```python
from build123d import *

# Parameters (mm, degrees)
CROQUIS1_R                        = 5.05
SALIENTE_EXTRUIR1_DEPTH           = 220
CORTAR_EXTRUIR1_REACH             = 7.05
CROQUIS2_R                        = 1.5
CORTAR_EXTRUIR1_DIRECTION_2_REACH = 7.05


with BuildPart() as part:
    # Croquis1 → Saliente-Extruir1 (new body)
    with BuildSketch(Plane(origin=(0, 0, 0), x_dir=(0, 0, -1), z_dir=(1, 0, 0))):
        Circle(CROQUIS1_R)
    extrude(amount=SALIENTE_EXTRUIR1_DEPTH)

    # Croquis2 → Cortar-Extruir1 (cut, up to next)
    with BuildSketch(Plane.XY, mode=Mode.PRIVATE) as cortar_extruir1_sk1:
        with Locations((3, 0)):
            Circle(CROQUIS2_R)
    cortar_extruir1_tool1 = extrude(cortar_extruir1_sk1.sketch, amount=-CORTAR_EXTRUIR1_REACH, mode=Mode.PRIVATE) & part.part
    add(cortar_extruir1_tool1.solids().sort_by_distance((3, 0, 0))[0], mode=Mode.SUBTRACT)
    # Croquis2 → Cortar-Extruir1 (cut, up to next)
    with BuildSketch(Plane.XY, mode=Mode.PRIVATE) as cortar_extruir1_sk2:
        with Locations((217, 0)):
            Circle(CROQUIS2_R)
    cortar_extruir1_tool2 = extrude(cortar_extruir1_sk2.sketch, amount=-CORTAR_EXTRUIR1_REACH, mode=Mode.PRIVATE) & part.part
    add(cortar_extruir1_tool2.solids().sort_by_distance((217, 0, 0))[0], mode=Mode.SUBTRACT)

    # Croquis2 → Cortar-Extruir1 direction 2 (cut, up to next)
    with BuildSketch(Plane.XY, mode=Mode.PRIVATE) as cortar_extruir1_direction_2_sk1:
        with Locations((3, 0)):
            Circle(CROQUIS2_R)
    cortar_extruir1_direction_2_tool1 = extrude(cortar_extruir1_direction_2_sk1.sketch, amount=CORTAR_EXTRUIR1_DIRECTION_2_REACH, mode=Mode.PRIVATE) & part.part
    add(cortar_extruir1_direction_2_tool1.solids().sort_by_distance((3, 0, 0))[0], mode=Mode.SUBTRACT)
    # Croquis2 → Cortar-Extruir1 direction 2 (cut, up to next)
    with BuildSketch(Plane.XY, mode=Mode.PRIVATE) as cortar_extruir1_direction_2_sk2:
        with Locations((217, 0)):
            Circle(CROQUIS2_R)
    cortar_extruir1_direction_2_tool2 = extrude(cortar_extruir1_direction_2_sk2.sketch, amount=CORTAR_EXTRUIR1_DIRECTION_2_REACH, mode=Mode.PRIVATE) & part.part
    add(cortar_extruir1_direction_2_tool2.solids().sort_by_distance((217, 0, 0))[0], mode=Mode.SUBTRACT)


solid = part.part
```
Geometry check sheet. Reference: the model listing, model coordinates, mm. Give positions to 0.01 mm unless a question says otherwise; leave off trailing zeros. Loops run counter-clockwise (first coordinate to the right, second up) from the corner with the lowest first, then second, coordinate; pieces in that order, holes last. Notation, with made-up numbers: (-21, 61.5) - (-4, 61.5) arc R27 ccw to (-4, 88.5) - close; hole circle Ø11 at (9, 82.5). An arc over 180 degrees is marked (long way). Use CSV: the item, a comma, the result in double quotes. Start each with the question number.
Q1. Go/stop test with flat-tipped pins: pin 1 Ø2 at (x, y) = (106, 1.5) entering from -Z; pin 2 Ø3 at (x, y) = (73.5, 3) entering from -Z. Record where each tip stops, or that it passes through.
Q2. Section check B-B, the plane x = 150. Record the cut outline in (y, z), and give its area (3 significant figures).
Q3. Scan lines: probe 1 along X at (y, z) = (-0.25, 2); probe 2 along Y at (x, z) = (217, 0.25); probe 3 along Y at (x, z) = (3, -1.75). Record each from-to range of solid material in increasing order. Write a range as from..to.
Q4. Section check A-A, the plane z = 3. Record the cut outline in (x, y), and give its area (3 significant figures).
Findings below:
1,pin 1,"stops at z = -5.03"
1,pin 2,"stops at z = -4.82"
2,outline,"circle Ø10.1 at (0, 0)"
2,area,"80.1 mm^2"
3,probe 1,"x = 0..1.52, 4.48..215.52, 218.48..220"
3,probe 2,"y = -5.04..-1.5, 1.5..5.04"
3,probe 3,"y = -4.74..-1.5, 1.5..4.74"
4,outline,"(0, -4.06) - (220, -4.06) - (220, 4.06) - (0, 4.06) - close; hole circle Ø3 at (3, 0); hole circle Ø3 at (217, 0)"
4,area,"1,770 mm^2"
